Input: part model. Units: mm. Frame: model coordinates. Round coordinates to 2 decimals unless told otherwise and drop trailing zeros. Use one line per item in the form item = value. Start each with the question number.
```python
from build123d import *

# Parameters (mm, degrees)
SKETCH1_R           = 1.5
BOSS_EXTRUDE1_DEPTH = 2
SKETCH4_R           = 14
SKETCH4_R_2         = 12
SKETCH4_R_3         = 10
CUT_EXTRUDE1_DEPTH  = 10


with BuildPart() as part:
    # Sketch1 → Boss-Extrude1 (new body)
    with BuildSketch(Plane.XY):
        with BuildLine():
            Line((60.447222151, 51.275649276), (51.275649276, 60.447222151))
            ThreePointArc((51.275649276, 60.447222151), (48.031415788, 62.614949665), (44.204581464, 63.376154339))
            add(Edge.make_bspline(
                [(-44.204581464, 63.376154339), (0, 53.376154339), (44.204581464, 63.376154339)],
                knots=[0, 0, 0, 1, 1, 1], degree=2))
            ThreePointArc((-44.204581464, 63.376154339), (-48.031415788, 62.614949665), (-51.275649276, 60.447222151))
            Line((-51.275649276, 60.447222151), (-60.447222151, 51.275649276))
            ThreePointArc((-60.447222151, 51.275649276), (-62.614949665, 48.031415788), (-63.376154339, 44.204581464))
            add(Edge.make_bspline(
                [(-63.376154339, -44.204581464), (-53.376154339, 0), (-63.376154339, 44.204581464)],
                knots=[0, 0, 0, 1, 1, 1], degree=2))
            ThreePointArc((-63.376154339, -44.204581464), (-62.614949665, -48.031415788), (-60.447222151, -51.275649276))
            Line((-60.447222151, -51.275649276), (-51.275649276, -60.447222151))
            ThreePointArc((-51.275649276, -60.447222151), (-48.031415788, -62.614949665), (-44.204581464, -63.376154339))
            add(Edge.make_bspline(
                [(44.204581464, -63.376154339), (0, -53.376154339), (-44.204581464, -63.376154339)],
                knots=[0, 0, 0, 1, 1, 1], degree=2))
            ThreePointArc((44.204581464, -63.376154339), (48.031415788, -62.614949665), (51.275649276, -60.447222151))
            Line((51.275649276, -60.447222151), (60.447222151, -51.275649276))
            ThreePointArc((60.447222151, -51.275649276), (62.614949665, -48.031415788), (63.376154339, -44.204581464))
            add(Edge.make_bspline(
                [(63.376154339, 44.204581464), (53.376154339, 0), (63.376154339, -44.204581464)],
                knots=[0, 0, 0, 1, 1, 1], degree=2))
            ThreePointArc((63.376154339, 44.204581464), (62.614949665, 48.031415788), (60.447222151, 51.275649276))
        make_face()
        with Locations((-47.376154339, -47.37615434)):
            Circle(SKETCH1_R, mode=Mode.SUBTRACT)
        with BuildLine():
            ThreePointArc((-28.761031711, -28.527510136), (-28.631586297, -28.644099888), (-28.51653182, -28.774911786))
            add(Edge.make_bspline(
                [(-21.191797917, -43.405881611), (-22.512426592, -34.921752495), (-28.516531822, -28.774911788)],
                knots=[0.024414386, 0.024414386, 0.024414386, 0.9806816, 0.9806816, 0.9806816], degree=2))
            ThreePointArc((-21.191797914, -43.40588161), (-21.143599518, -43.62088039), (-21.127416998, -43.840620434))
            ThreePointArc((-21.127416998, -43.840620434), (-22.627416998, -45.340620434), (-24.127416998, -43.840620434))
            add(Edge.make_bspline(
                [(-24.127416998, -43.840620434), (-25.362407372, -36.251653189), (-30.759144982, -30.759144982)],
                knots=[0, 0, 0, 1, 1, 1], degree=2))
            ThreePointArc((-30.759144982, -30.759144982), (-30.816001484, -28.697906735), (-28.761031711, -28.527510136))
        make_face(mode=Mode.SUBTRACT)
        with BuildLine():
            add(Edge.make_bspline(
                [(24.127416998, -43.840620434), (25.362407372, -36.251653189), (30.759144982, -30.759144982)],
                knots=[0, 0, 0, 1, 1, 1], degree=2))
            ThreePointArc((24.127416998, -43.840620434), (22.627416998, -45.340620434), (21.127416998, -43.840620434))
            ThreePointArc((21.127416998, -43.840620434), (21.143599518, -43.62088039), (21.191797914, -43.40588161))
            add(Edge.make_bspline(
                [(21.191797917, -43.405881611), (22.512426592, -34.921752495), (28.516531822, -28.774911788)],
                knots=[0.024414386, 0.024414386, 0.024414386, 0.9806816, 0.9806816, 0.9806816], degree=2))
            ThreePointArc((28.51653182, -28.774911786), (28.631586297, -28.644099888), (28.761031711, -28.527510136))
            ThreePointArc((28.761031711, -28.527510136), (30.816001484, -28.697906735), (30.759144982, -30.759144982))
        make_face(mode=Mode.SUBTRACT)
        with Locations((47.376154339, -47.376154339)):
            Circle(SKETCH1_R, mode=Mode.SUBTRACT)
        with Locations((-47.376154339, 47.376154339)):
            Circle(SKETCH1_R, mode=Mode.SUBTRACT)
        with BuildLine():
            add(Edge.make_bspline(
                [(-24.127416998, 43.840620434), (-25.362407372, 36.251653189), (-30.759144982, 30.759144982)],
                knots=[0, 0, 0, 1, 1, 1], degree=2))
            ThreePointArc((-24.127416998, 43.840620434), (-22.627416998, 45.340620434), (-21.127416998, 43.840620434))
            ThreePointArc((-21.127416998, 43.840620434), (-21.143599518, 43.62088039), (-21.191797914, 43.40588161))
            add(Edge.make_bspline(
                [(-21.191797917, 43.405881611), (-22.512426592, 34.921752495), (-28.516531822, 28.774911788)],
                knots=[0.024414386, 0.024414386, 0.024414386, 0.9806816, 0.9806816, 0.9806816], degree=2))
            ThreePointArc((-28.51653182, 28.774911786), (-28.631586297, 28.644099888), (-28.761031711, 28.527510136))
            ThreePointArc((-28.761031711, 28.527510136), (-30.816001484, 28.697906735), (-30.759144982, 30.759144982))
        make_face(mode=Mode.SUBTRACT)
        with BuildLine():
            ThreePointArc((28.761031711, 28.527510136), (28.631586297, 28.644099888), (28.51653182, 28.774911786))
            add(Edge.make_bspline(
                [(23.673604803, 35.525452482), (25.506528794, 31.856471559), (28.516531822, 28.774911788)],
                knots=[0.501281739, 0.501281739, 0.501281739, 0.9806816, 0.9806816, 0.9806816], degree=2))
            add(Edge.make_bspline(
                [(21.191797917, 43.405881611), (21.850363527, 39.175051421), (23.673604803, 35.525452482)],
                knots=[0.024414386, 0.024414386, 0.024414386, 0.501281739, 0.501281739, 0.501281739], degree=2))
            ThreePointArc((21.191797914, 43.40588161), (21.143599518, 43.62088039), (21.127416998, 43.840620434))
            ThreePointArc((21.127416998, 43.840620434), (22.627416998, 45.340620434), (24.127416998, 43.840620434))
            add(Edge.make_bspline(
                [(24.127416998, 43.840620434), (24.734971072, 40.107224563), (26.349731434, 36.881203745)],
                knots=[0, 0, 0, 0.491950453, 0.491950453, 0.491950453], degree=2))
            ThreePointArc((26.349731434, 36.881203745), (26.356395509, 36.86807251), (26.362930356, 36.854876488))
            add(Edge.make_bspline(
                [(26.362930356, 36.854876488), (28.028171669, 33.538582193), (30.759144982, 30.759144982)],
                knots=[0.493958478, 0.493958478, 0.493958478, 1, 1, 1], degree=2))
            ThreePointArc((30.759144982, 30.759144982), (30.816001484, 28.697906735), (28.761031711, 28.527510136))
        make_face(mode=Mode.SUBTRACT)
        with Locations((47.376154339, 47.376154339)):
            Circle(SKETCH1_R, mode=Mode.SUBTRACT)
    extrude(amount=BOSS_EXTRUDE1_DEPTH)

    # Sketch4 → Cut-Extrude1 (cut)
    with BuildSketch(Plane(origin=(0, 0, 0), x_dir=(-1, 0, 0), z_dir=(0, 0, -1))):
        Circle(SKETCH4_R)
        with Locations((-36, 0)):
            Circle(SKETCH4_R_2)
        with Locations((36, 0)):
            Circle(SKETCH4_R_2)
        with Locations((0, 35)):
            Circle(SKETCH4_R_3)
        with Locations((0, -35)):
            Circle(SKETCH4_R_3)
        with BuildLine():
            Line((-8.965692962, 20), (8.965692962, 20))
            ThreePointArc((8.965692962, 20), (10.965692962, 18), (8.965692962, 16))
            Line((8.965692962, 16), (-8.965692962, 16))
            ThreePointArc((-8.965692962, 16), (-10.965692962, 18), (-8.965692962, 20))
        make_face()
        with BuildLine():
            Line((8.965692962, -20), (-8.965692962, -20))
            ThreePointArc((-8.965692962, -20), (-10.965692962, -18), (-8.965692962, -16))
            Line((-8.965692962, -16), (8.965692962, -16))
            ThreePointArc((8.965692962, -16), (10.965692962, -18), (8.965692962, -20))
        make_face()
    extrude(amount=-CUT_EXTRUDE1_DEPTH, mode=Mode.SUBTRACT)


solid = part.part
```
Item 1: Draft query along Y for faces 1 (the face through (-55.926, -55.797, 0.986)), 2 (the face through (48.18, -46.11, 0.99)), 3 (the face through (-15, 1, 0)). Return one class per face: +Y half, -Y half, draft (parallel to the pull), parting line (faces both ways), or undercut.
Item 2: First-contact query: pin 1 (1 mm diameter, centred on y = -46.5, z = 1.5, fed in from +X). Flat tip, straight axial feed; report the tip coordinate or a pass-through.
Item 3: Ray query, line 1 (Y direction, x = 0, z = 1.4); line 2 (Y direction, x = 23, z = 1.9); line 3 (Y direction, x = 48.5, z = 1.45). Return the intervals inside material, ascending. Write a range as from..to.
Item 4: Cut plane A-A (x = 0). Give the number of separate pieces and of enclosed holes in the cut face, plus the area to 3 significant figures.
Final values:
q1.face_1 = -Y half
q1.face_2 = undercut
q1.face_3 = draft
q2.pin_1 = 63.21
q3.line_1 = -58.38..-45, -25..-20, -16..-14, 14..16, 20..25, 45..58.38
q3.line_2 = -59.73..-45.29, -36.99..36.99, 45.29..59.73
q3.line_3 = -62.41..-48.37, -46.38..46.38, 48.37..62.41
q4.separate_pieces = 6
q4.enclosed_holes = 0
q4.area = 81.5 mm^2
